Design review of the part built by this model. Coordinates are the model's own, in mm. Round coordinates to 2 decimals unless told otherwise and drop trailing zeros. Write item = value, one per line. Start each with the question number.
Item 1: To check wall thickness, follow L1, parallel to Z at x = 2.5, y = -0.5; L2, parallel to Z at x = 3.5, y = -1.25; L3, parallel to X at y = -1, z = 5. State the ranges of each line that lie inside material, in increasing order.
Item 2: For pin 1 Ø3 at (y, z) = (-3, 47) entering from -X; pin 2 Ø2 at (x, y) = (2, -1.5) entering from -Z, all flat-tipped, find the tip position at first contact; note any pin that passes through.
Item 3: Add section A-A, the plane x = 3. State how many separate pieces and enclosed holes the cut face has, then the cut area to 3 significant figures.
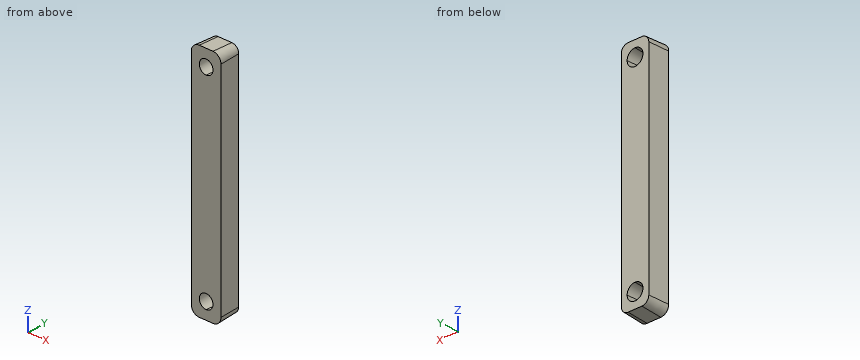
from build123d import *

# Parameters (mm, degrees)
F1_DEPTH = 6
F1_TAPER = -3


with BuildPart() as f1:
    # F0 (on Front) → F1 (new body)
    with BuildSketch(Plane.XZ):
        with BuildLine():
            ThreePointArc((0, 2), (0.5857864376, 0.5857864376), (2, 0))
            Line((2, 0), (4, 0))
            Line((4, 0), (4, 2))
            ThreePointArc((4, 2), (1.7, 4.3), (4, 6.6))
            Line((4, 6.6), (4, 59.5))
            ThreePointArc((4, 59.5), (1.7, 61.8), (4, 64.1))
            Line((4, 64.1), (4, 66.1))
            Line((4, 66.1), (2, 66.1))
            ThreePointArc((2, 66.1), (0.5857864376, 65.5142135624), (0, 64.1))
            Line((0, 64.1), (0, 2))
        make_face()
        with BuildLine():
            Line((4, 2), (4, 0))
            Line((4, 0), (6, 0))
            ThreePointArc((6, 0), (7.4142135624, 0.5857864376), (8, 2))
            Line((8, 2), (8, 64.1))
            ThreePointArc((8, 64.1), (7.4142135624, 65.5142135624), (6, 66.1))
            Line((6, 66.1), (4, 66.1))
            Line((4, 66.1), (4, 64.1))
            ThreePointArc((4, 64.1), (5.6263455967, 63.4263455967), (6.3, 61.8))
            ThreePointArc((6.3, 61.8), (5.6263455967, 60.1736544033), (4, 59.5))
            Line((4, 59.5), (4, 6.6))
            ThreePointArc((4, 6.6), (5.6263455967, 5.9263455967), (6.3, 4.3))
            ThreePointArc((6.3, 4.3), (5.6263455967, 2.6736544033), (4, 2))
        make_face()
    extrude(amount=F1_DEPTH, taper=F1_TAPER)


solid = f1.part
Result set:
q1.L1 = -0.03 to 2.59, 6.01 to 60.09, 63.51 to 66.13
q1.L2 = -0.07 to 2.12, 6.48 to 59.62, 63.98 to 66.17
q1.L3 = -0.05 to 1.86, 6.14 to 8.05
q2.pin_1 = -0.24
q2.pin_2 = -0.13
q3.separate_pieces = 3
q3.enclosed_holes = 0
q3.area = 353 mm²
